Check sheet for the modelled part. Datum: model origin and axes. Units: mm. A direction names the side the tool comes from. Coordinates: 2 decimals unless noted, no trailing zeros. Loops run counter-clockwise (first coordinate to the right, second up) from the corner with the lowest first, then second, coordinate; pieces in that order, holes last. Notation, with made-up numbers: (49, 41) - (89, 41) arc R18 cw to (89, 68) - close; hole circle Ø8 at (29.25, 89). An arc over 180 degrees is marked (long way). Answer as a JSON object with one key per item and string values. Group by question number.
from build123d import *

# Parameters (mm, degrees)
F0_R      = 9
F1_DEPTH  = 65
F2_W      = 23
F2_H      = 36
F2_H_2    = 3
F3_DEPTH  = 72
F4_R      = 12
F5_DEPTH  = 4
F6_R      = 27
F7_DEPTH  = 23
F8_R      = 12
F9_DEPTH  = 10
F11_DEPTH = 6
F13_DEPTH = 65


with BuildPart() as f1:
    # F0 (on Front) → F1 (new body)
    with BuildSketch(Plane.XZ):
        with BuildLine():
            Line((36, -37), (36, 0))
            ThreePointArc((36, 0), (0, 36), (-36, 0))
            Line((-36, 0), (-36, -37))
            Line((-36, -37), (36, -37))
        make_face()
        Circle(F0_R, mode=Mode.SUBTRACT)
    extrude(amount=-F1_DEPTH)

    # F2 (on face) → F3 (cut)
    with BuildSketch(Plane.YZ.offset(36)):
        with Locations((53.5, 18)):
            Rectangle(F2_W, F2_H)
        with Locations((53.5, -1.5)):
            Rectangle(F2_W, F2_H_2)
    extrude(amount=-F3_DEPTH, mode=Mode.SUBTRACT)

    # F4 (on face) → F5 (cut)
    with BuildSketch(Plane.XZ):
        Circle(F4_R)
    extrude(amount=-F5_DEPTH, mode=Mode.SUBTRACT)

    # F6 (on face) → F7 (cut)
    with BuildSketch(Plane(origin=(0, 65, 0), x_dir=(-1, 0, 0), z_dir=(0, 1, 0))):
        Circle(F6_R)
    extrude(amount=-F7_DEPTH, mode=Mode.SUBTRACT)

    # F8 (on face) → F9 (cut)
    with BuildSketch(Plane(origin=(0, 42, 0), x_dir=(-1, 0, 0), z_dir=(0, 1, 0))):
        Circle(F8_R)
    extrude(amount=-F9_DEPTH, mode=Mode.SUBTRACT)

    # F10 (on face) → F11 (cut)
    with BuildSketch(Plane(origin=(0, 42, 0), x_dir=(-1, 0, 0), z_dir=(0, 1, 0))):
        with BuildLine():
            ThreePointArc((22.1415898255, 0), (25.2111536743, 1.4352821251), (26.0778724611, 4.7111111111))
            ThreePointArc((26.0778724611, 4.7111111111), (0, 26.5), (-26.0778724611, 4.7111111111))
            ThreePointArc((-26.0778724611, 4.7111111111), (-25.2111536743, 1.4352821251), (-22.1415898255, 0))
            Line((-22.1415898255, 0), (22.1415898255, 0))
        make_face()
    extrude(amount=-F11_DEPTH, mode=Mode.SUBTRACT)

    # F12 (on face) → F13 (cut)
    with BuildSketch(Plane.XZ):
        with BuildLine():
            ThreePointArc((19.8995, 30.0001649954), (0, 36), (-19.8995, 30.0001649954))
            Line((-19.8995, 30.0001649954), (19.8995, 30.0001649954))
        make_face()
    extrude(amount=-F13_DEPTH, mode=Mode.SUBTRACT)


solid = f1.part
1. Release check for a two-part mould opening along Z. For faces 6 (the face through (36, 32, -19)), 7 (the face through (-31.602, 20.706, 17.242)), 8 (the face through (-0.516, 39.042, 26.495)) record: released by +Z, released by -Z, zero draft, split by the parting line, or undercut.
2. Sectioned sample at B-B on x = 0. Record the cut outline in (y, z).
3. Gauge pin test, flat ends, axial feed: pin 1 (14.5 mm diameter, centred on x = 0, z = 0, fed in from -Y); pin 2 (5 mm diameter, centred on x = 2.5, y = 50, fed in from +Z); pin 3 (1.5 mm diameter, centred on y = 37.5, z = 11.5, fed in from -X); pin 4 (10 mm diameter, centred on x = 31, y = 52.5, fed in from +Z). Record the tip position at first contact, or that the pin passes through.
4. Material ranges on line 1 (Z direction, x = 0, y = 38); line 2 (Z direction, x = 0, y = 16.75); line 3 (Z direction, x = 1, y = 52.5), recorded low to high.
5. Access from +Z, -Z, +X, -X, +Y, -Y to the whole of each face (thin tool, end or side, straight path). Record for faces 1 (the face through (-7, 42, -11)), 2 (the face through (-11.99, 1.97, 0.53)), 3 (the face through (-31, 53, -3)), 4 (the face through (0, 36, 13)), 5 (the face through (31.84, 20.71, 16.8)).
6. Sectioned sample at D-D on z = -24.5. Record the cut outline in (x, y).
7. Sectioned sample at C-C on y = 8. Record the cut outline in (x, z), plus the area to 3 significant figures.
8. Sectioned sample at A-A on y = 40.5. Record the cut outline in (x, z).
Answers follow:
{
 "1": {"face 6": "zero draft", "face 7": "released by +Z", "face 8": "undercut"},
 "2": {"outline": "(0, -37) - (65, -37) - (65, -27) - (42, -27) - (42, -12) - (32, -12) - (32, -9) - (4, -9) - (4, -12) - (0, -12) - close; (0, 12) - (4, 12) - (4, 9) - (32, 9) - (32, 12) - (36, 12) - (36, 26.5) - (42, 26.5) - (42, 30) - (0, 30) - close"},
 "3": {"pin 1": "passes through", "pin 2": "stops at z = -26.53", "pin 3": "stops at x = -34.36", "pin 4": "stops at z = -3"},
 "4": {"line 1": "z = -37 to -12, 26.5 to 30", "line 2": "z = -37 to -9, 9 to 30", "line 3": "z = -37 to -26.98"},
 "5": {"face 1": "+Z, +Y", "face 2": "-Y", "face 3": "+Z, +X, -X, +Y", "face 4": "+Y", "face 5": "+Z, +X, +Y, -Y"},
 "6": {"outline": "(-36, 0) - (36, 0) - (36, 65) - (11.35, 65) - (11.35, 42) - (-11.35, 42) - (-11.35, 65) - (-36, 65) - close"},
 "7": {"outline": "(-36, -37) - (36, -37) - (36, 0) arc R36 ccw to (19.9, 30) - (-19.9, 30) arc R36 ccw to (-36, 0) - close; hole circle Ø18 at (0, 0)", "area": "4,280 mm^2"},
 "8": {"outline": "(-36, -37) - (36, -37) - (36, 0) arc R36 ccw to (19.9, 30) - (-19.9, 30) arc R36 ccw to (-36, 0) - close; hole (-26.08, 4.71) arc R4 ccw to (-22.14, 0) - (-12, 0) arc R12 ccw to (12, 0) - (22.14, 0) arc R4 ccw to (26.08, 4.71) arc R26.5 ccw to start"}
}
